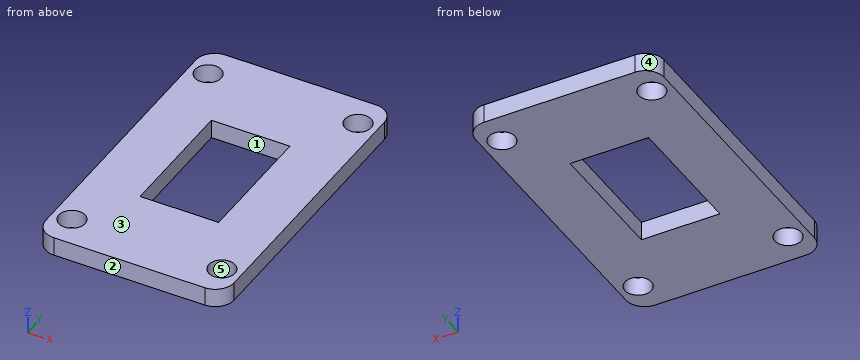
from build123d import *

# Parameters (mm, degrees)
SKETCH1_W           = 30
SKETCH1_H           = 48.96
SKETCH1_R           = 2.1
SKETCH1_W_2         = 12.5
SKETCH1_H_2         = 20.4
BOSS_EXTRUDE1_DEPTH = 3
FILLET1_R           = 3


with BuildPart() as part:
    # Sketch1 → Boss-Extrude1 (new body)
    with BuildSketch(Plane.XY):
        Rectangle(SKETCH1_W, SKETCH1_H)
        with Locations((-11.93627451, 19.48)):
            Circle(SKETCH1_R, mode=Mode.SUBTRACT)
        with Locations((11.93627451, 19.48)):
            Circle(SKETCH1_R, mode=Mode.SUBTRACT)
        with Locations((11.93627451, -19.48)):
            Circle(SKETCH1_R, mode=Mode.SUBTRACT)
        with Locations((-11.93627451, -19.48)):
            Circle(SKETCH1_R, mode=Mode.SUBTRACT)
        Rectangle(SKETCH1_W_2, SKETCH1_H_2, mode=Mode.SUBTRACT)
    extrude(amount=BOSS_EXTRUDE1_DEPTH)

    # Fillet1
    fillet1_edges = [part.edges().sort_by_distance(p)[0] for p in [
        (15, -24.48, 1.5),
        (-15, -24.48, 1.5),
        (-15, 24.48, 1.5),
        (15, 24.48, 1.5),
    ]]
    fillet(fillet1_edges, radius=FILLET1_R)


solid = part.part
Source: CAD feature listing. Evaluate the final solid. Frame: model axes, mm. Face numbers are marked on the shaded views. A direction names the side the tool comes from. Coordinates: 2 decimals unless noted, no trailing zeros. Write each loop counter-clockwise with the first axis right and the second up, starting at its lowest first coordinate (ties: lowest second). Pieces come first, ordered by that corner, then holes. Notation, with made-up numbers: M 10,-10 L 56,-10 A22 ccw 56,27 Z; hole C 21,31 d4. An arc over 180 degrees is marked long. Use a Markdown table: item, result.
1) Section A-A, the plane y = -4. Output: boundary loops of the cut face in (x, z), then the cut area to 3 significant figures.
Conclusion:
| item | result |
|---|---|
| outline | M -15,0 L -6.25,0 L -6.25,3 L -15,3 Z; M 6.25,0 L 15,0 L 15,3 L 6.25,3 Z |
| area | 52.5 mm^2 |
2) Mould query, pull axis X, two halves, no side actions, for the marked faces 3, 4 and 5. Classes: pulls with the +X half, pulls with the -X half, needs draft (parallel to the pull), parting line crosses it, or undercut.
Conclusion:
| item | result |
|---|---|
| face 3 | needs draft |
| face 4 | pulls with the -X half |
| face 5 | undercut |
3) Section C-C, the plane y = 19.48. Output: boundary loops of the cut face in (x, z).
Conclusion:
| item | result |
|---|---|
| outline | M -15,0 L -14.04,0 L -14.04,3 L -15,3 Z; M -9.84,0 L 9.84,0 L 9.84,3 L -9.84,3 Z; M 14.04,0 L 15,0 L 15,3 L 14.04,3 Z |
4) Section B-B, the plane z = 2.1. Output: boundary loops of the cut face in (x, y), then the cut area to 3 significant figures.
Conclusion:
| item | result |
|---|---|
| outline | M -15,-21.48 A3 ccw -12,-24.48 L 12,-24.48 A3 ccw 15,-21.48 L 15,21.48 A3 ccw 12,24.48 L -12,24.48 A3 ccw -15,21.48 Z; hole C -11.94,-19.48 d4.2; hole C -11.94,19.48 d4.2; hole M -6.25,-10.2 L 6.25,-10.2 L 6.25,10.2 L -6.25,10.2 Z; hole C 11.94,-19.48 d4.2; hole C 11.94,19.48 d4.2 |
| area | 1,150 mm^2 |
5) First-contact query: pin 1 Ø6.5 at (x, y) = (11.94, -19.48) entering from +Z. Flat tip, straight axial feed; report the tip coordinate or a pass-through.
Conclusion:
| item | result |
|---|---|
| pin 1 | stops at z = 3 |
6) Ray query, L1, parallel to Y at x = -11.75, z = 0.8; L2, parallel to X at y = -7, z = 1.15; L3, parallel to Y at x = -2.25, z = 2.15. Return the intervals inside material, ascending.
Conclusion:
| item | result |
|---|---|
| L1 | y = -24.48 to -21.57, -17.39 to 17.39, 21.57 to 24.48 |
| L2 | x = -15 to -6.25, 6.25 to 15 |
| L3 | y = -24.48 to -10.2, 10.2 to 24.48 |
7) Section D-D, the plane x = -2. Output: boundary loops of the cut face in (y, z), then the cut area to 3 significant figures.
Conclusion:
| item | result |
|---|---|
| outline | M -24.48,0 L -10.2,0 L -10.2,3 L -24.48,3 Z; M 10.2,0 L 24.48,0 L 24.48,3 L 10.2,3 Z |
| area | 85.7 mm^2 |
8) Reachability of the marked faces 1 and 2 from +Z, -Z, +X, -X, +Y, -Y: full face, straight path, thin tool, end or side. Return the list, or none.
Conclusion:
| item | result |
|---|---|
| face 1 | +Z, -Z |
| face 2 | +Z, -Z, +X, -X, -Y |
